```python
from build123d import *

# Parameters (mm, degrees)
SKETCH_1_R         = 3
EXTRUDE_1_DEPTH    = 10
HOLE_WIZARD_M3_1_D = 2.5
CHAMFER_1_SIZE     = 0.2


with BuildPart() as part:
    # 草图1 → 凸台-拉伸1 (new body)
    with BuildSketch(Plane.XY):
        Circle(SKETCH_1_R)
    extrude(amount=EXTRUDE_1_DEPTH)

    # M3 螺纹孔1 (through all)
    with Locations(Plane.XY.offset(10)):
        with Locations((0, 0)):
            Hole(HOLE_WIZARD_M3_1_D / 2)

    # 倒角1
    chamfer_1_edges = [part.edges().sort_by_distance(p)[0] for p in [
        (-3, 0, 10),
        (1.25, 0, 10),
        (1.25, 0, 0),
    ]]
    chamfer(chamfer_1_edges, length=CHAMFER_1_SIZE)


solid = part.part
```
The listing builds one solid part. Answer for the finished solid, in the listing's coordinates (mm). Coordinates: 2 decimals unless noted, no trailing zeros. Loops run counter-clockwise (first coordinate to the right, second up) from the corner with the lowest first, then second, coordinate; pieces in that order, holes last. Notation, with made-up numbers: (6, -22.5) -> (34, -22.5) arc R30 ccw to (34, -0.5) -> close; hole circle Ø5 at (-32, 22.25). An arc over 180 degrees is marked (long way). Return JSON: item names as keys, results as strings. Group by question number.
(1) Find the intervals of material crossed by probe 1 along Y at (x, z) = (0, 6.75); probe 2 along Y at (x, z) = (-0.9, 3.5); probe 3 along X at (y, z) = (0.75, 4.75), in increasing order. Write a range as from..to.
(2) A cutting plane is placed at C-C on z = 9. Write down the section's boundary in (x, y), and give its area (3 significant figures).
(3) A cutting plane is placed at A-A on y = 0. Write down the section's boundary in (x, z), and give its area (3 significant figures).
(4) Determine the mould class of faces 1 (the cylindrical face through (0.27, -1.22, 4.93)), 2 (the flat face through (1.2, -1.2, 10)), 3 (the cylindrical face through (-3, 0, 5)) for opening direction Y: released by +Y, released by -Y, zero draft, split by the parting line, or undercut.
The answers:
{
 "1": {"probe 1": "y = -3..-1.25, 1.25..3", "probe 2": "y = -2.86..-0.87, 0.87..2.86", "probe 3": "x = -2.9..-1, 1..2.9"},
 "2": {"outline": "circle Ø6 at (0, 0); hole circle Ø2.5 at (0, 0)", "area": "23.4 mm^2"},
 "3": {"outline": "(-3, 0) -> (-1.45, 0) -> (-1.25, 0.2) -> (-1.25, 9.8) -> (-1.45, 10) -> (-2.8, 10) -> (-3, 9.8) -> close; (1.25, 0.2) -> (1.45, 0) -> (3, 0) -> (3, 9.8) -> (2.8, 10) -> (1.45, 10) -> (1.25, 9.8) -> close", "area": "34.9 mm^2"},
 "4": {"face 1": "undercut", "face 2": "zero draft", "face 3": "split by the parting line"}
}
